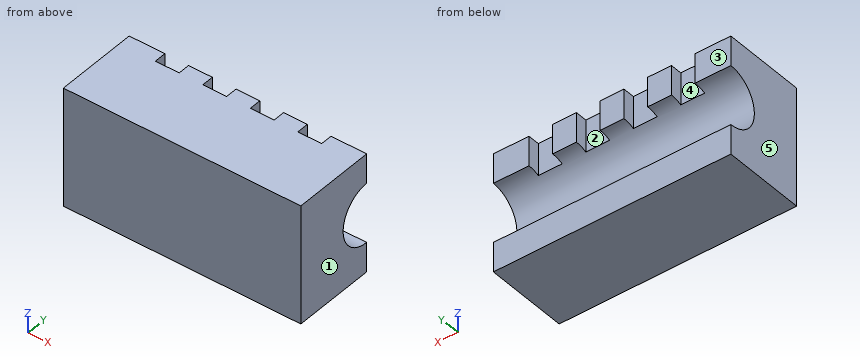
from build123d import *

# Parameters (mm, degrees)
SKETCH1_W           = 100
SKETCH1_H           = 50
BOSS_EXTRUDE1_DEPTH = 35
SKETCH2_R           = 12.5
CUT_EXTRUDE1_DEPTH  = 100
SKETCH5_W           = 10
SKETCH5_H           = 5
CUT_EXTRUDE3_DEPTH  = 25


with BuildPart() as part:
    # Sketch1 → Boss-Extrude1 (new body)
    with BuildSketch(Plane(origin=(0, 0, 0), x_dir=(1, 0, 0), z_dir=(0, 1, 0))):
        with Locations((50, 25)):
            Rectangle(SKETCH1_W, SKETCH1_H)
    extrude(amount=BOSS_EXTRUDE1_DEPTH)

    # Sketch2 → Cut-Extrude1 (cut)
    with BuildSketch(Plane(origin=(100, 0, 0), x_dir=(0, 0, -1), z_dir=(1, 0, 0))):
        with Locations((25, 35)):
            Circle(SKETCH2_R)
    extrude(amount=-CUT_EXTRUDE1_DEPTH, mode=Mode.SUBTRACT)

    # Sketch5 → Cut-Extrude3 (cut)
    with BuildSketch(Plane.XY):
        with Locations((20, 32.5)):
            Rectangle(SKETCH5_W, SKETCH5_H)
        with Locations((40, 32.5)):
            Rectangle(SKETCH5_W, SKETCH5_H)
        with Locations((60, 32.5)):
            Rectangle(SKETCH5_W, SKETCH5_H)
        with Locations((80, 32.5)):
            Rectangle(SKETCH5_W, SKETCH5_H)
    extrude(amount=-CUT_EXTRUDE3_DEPTH, mode=Mode.SUBTRACT)


solid = part.part
Can you work these out from the model? Positions are in its coordinate system, mm. Face numbers are marked on the shaded views. A direction names the side the tool comes from. Coordinates: 2 decimals unless noted, no trailing zeros. Write each loop counter-clockwise with the first axis right and the second up, starting at its lowest first coordinate (ties: lowest second). Pieces come first, ordered by that corner, then holes. Notation, with made-up numbers: (65, 72) - (96, 72) arc R20 ccw to (96, 103) - close; hole circle Ø7 at (77, 84.25). An arc over 180 degrees is marked (long way). Return JSON: item names as keys, results as strings. Group by question number.
Item 1: If we section it at A-A (x = 73): Write out the boundary of the cut face in (y, z), then the cut area to 3 significant figures.
Item 2: We'd pull the mould along X, two halves only. Please class the marked faces 1, 2 and 3: pulls with the +X half, pulls with the -X half, needs draft (parallel to the pull), parting line crosses it, or undercut.
Item 3: If we section it at D-D (z = -25): Write out the boundary of the cut face in (x, y), then the cut area to 3 significant figures.
Item 4: If we section it at B-B (z = -4): Write out the boundary of the cut face in (x, y).
Item 5: Please list where these lines run through material, in increasing order: probe 1 along Z at (x, y) = (23.5, 23.5); probe 2 along Z at (x, y) = (61, 25); probe 3 along Y at (x, z) = (15.5, -4).
Item 6: Which directions (+Z, -Z, +X, -X, +Y, -Y) give clear straight access to the entire face, cutting with the end or side of a thin tool? Please do the marked faces 4 and 5.
Item 7: I'm going to push flat-ended pins straight in: pin 1 Ø2.5 at (y, z) = (33.5, -7) entering from -X; pin 2 Ø3 at (x, z) = (80.5, -4) entering from +Y; pin 3 Ø2 at (x, z) = (79, -28.5) entering from +Y; pin 4 Ø2 at (x, z) = (29.5, -26) entering from +Y. Where does each tip first touch, or does it pass through?
Item 8: If we section it at C-C (x = 20.5): Write out the boundary of the cut face in (y, z), then the cut area to 3 significant figures.
Return value:
{
 "1": {"outline": "(0, -50) - (35, -50) - (35, -37.5) arc R12.5 cw to (35, -12.5) - (35, 0) - (0, 0) - close", "area": "1,500 mm^2"},
 "2": {"face 1": "pulls with the +X half", "face 2": "undercut", "face 3": "needs draft"},
 "3": {"outline": "(0, 0) - (100, 0) - (100, 22.5) - (0, 22.5) - close", "area": "2,250 mm^2"},
 "4": {"outline": "(0, 0) - (100, 0) - (100, 35) - (85, 35) - (85, 30) - (75, 30) - (75, 35) - (65, 35) - (65, 30) - (55, 30) - (55, 35) - (45, 35) - (45, 30) - (35, 30) - (35, 35) - (25, 35) - (25, 30) - (15, 30) - (15, 35) - (0, 35) - close"},
 "5": {"probe 1": "z = -50 to -29.9, -20.1 to 0", "probe 2": "z = -50 to -32.5, -17.5 to 0", "probe 3": "y = 0 to 30"},
 "6": {"face 4": "+Z, +Y", "face 5": "+Z, -Z, -X, +Y, -Y"},
 "7": {"pin 1": "stops at x = 0", "pin 2": "stops at y = 30", "pin 3": "stops at y = 23.34", "pin 4": "stops at y = 22.66"},
 "8": {"outline": "(0, -50) - (35, -50) - (35, -37.5) arc R12.5 cw to (30, -13.54) - (30, 0) - (0, 0) - close", "area": "1,440 mm^2"}
}
